Here's how the part is built. I have some questions about the finished solid (model axes, mm). A direction names the side the tool comes from. Give positions to 0.01 mm unless a question says otherwise; leave off trailing zeros. Order: outer loops, then holes, each group sorted by start corner. A loop starts at its lowest first (then second) coordinate and runs counter-clockwise, first axis right, second up. Notation, with made-up numbers: M -1.5,32 L 15.5,32 A24 cw 15.5,55 Z; hole C 40.5,66 d9. An arc over 180 degrees is marked long. Use CSV: the item, a comma, the result in double quotes. Start each with the question number.
```python
from build123d import *

# Parameters (mm, degrees)
PAD028_DEPTH            = 9
SKETCH075_R             = 11.25
POCKET028_DEPTH         = 7
SKETCH076_R             = 8
POCKET029_DEPTH         = 5
SKETCH077_W             = 16
SKETCH077_H             = 37
PAD029_DEPTH            = 9
SKETCH078_W             = 14
SKETCH078_H             = 35
POCKET030_DEPTH         = 1
SKETCH079_W             = 12
SKETCH079_H             = 33
POCKET031_DEPTH         = 5
SKETCH080_W             = 10
SKETCH080_H             = 4
POCKET032_DEPTH         = 5
HOLE007_D               = 4.5
HOLE007_DEPTH           = 25
HOLE007_CBORE_D         = 7.5
HOLE007_CBORE_DEPTH     = 4
FILLET006_R             = 2
BODY010_ROLL_ANGLE      = 180
BODY010_PLACEMENT_ANGLE = -90


with BuildPart() as part:
    # Sketch074 → Pad028 (new body)
    with BuildSketch(Plane.XY):
        with BuildLine():
            ThreePointArc((12.269609, 5), (-13.250782, 0), (12.269609, -5))
            Line((12.269609, -5), (47.729609, -5))
            ThreePointArc((47.729609, -5), (73.25, 0), (47.729609, 5))
            Line((12.269609, 5), (47.729609, 5))
        make_face()
    extrude(amount=PAD028_DEPTH)

    # Sketch075 (on Face6 of Pad028) → Pocket028 (cut)
    with BuildSketch(Plane.XY.offset(9)):
        Circle(SKETCH075_R)
        with Locations((60, 0)):
            Circle(SKETCH075_R)
    extrude(amount=-POCKET028_DEPTH, mode=Mode.SUBTRACT)

    # Sketch076 (on Face4 of Pocket028) → Pocket029 (cut)
    with BuildSketch(Plane(origin=(0, 0, 0), x_dir=(1, 0, 0), z_dir=(0, 0, -1))):
        Circle(SKETCH076_R)
        with Locations((60, 0)):
            Circle(SKETCH076_R)
    extrude(amount=-POCKET029_DEPTH, mode=Mode.SUBTRACT)

    # Sketch077 (on Face4 of Pocket029) → Pad029 (join)
    with BuildSketch(Plane(origin=(0, 0, 0), x_dir=(1, 0, 0), z_dir=(0, 0, -1))):
        with Locations((30, -4.5)):
            Rectangle(SKETCH077_W, SKETCH077_H)
    extrude(amount=-PAD029_DEPTH)

    # Sketch078 (on Face13 of Pad029) → Pocket030 (cut)
    with BuildSketch(Plane.XY.offset(9)):
        with Locations((30, 4.5)):
            Rectangle(SKETCH078_W, SKETCH078_H)
    extrude(amount=-POCKET030_DEPTH, mode=Mode.SUBTRACT)

    # Sketch079 (on Face22 of Pocket030) → Pocket031 (cut)
    with BuildSketch(Plane.XY.offset(9)):
        with Locations((30, 4.5)):
            Rectangle(SKETCH079_W, SKETCH079_H)
    extrude(amount=-POCKET031_DEPTH, mode=Mode.SUBTRACT)

    # Sketch080 (on Face14 of Pocket031) → Pocket032 (cut)
    with BuildSketch(Plane(origin=(0, 23, 0), x_dir=(-1, 0, 0), z_dir=(0, 1, 0))):
        with Locations((-30, 5)):
            Rectangle(SKETCH080_W, SKETCH080_H)
    extrude(amount=-POCKET032_DEPTH, mode=Mode.SUBTRACT)

    # Hole007
    with Locations(Plane(origin=(0, 0, 0), x_dir=(1, 0, 0), z_dir=(0, 0, -1))):
        with Locations((17, 0), (43, 0)):
            CounterBoreHole(HOLE007_D / 2, HOLE007_CBORE_D / 2, HOLE007_CBORE_DEPTH, depth=HOLE007_DEPTH)

    # Fillet006
    fillet006_edges = [part.edges().sort_by_distance(p)[0] for p in [
        (38, 23, 4.5),
        (22, 23, 4.5),
        (22, -14, 4.5),
        (38, -14, 4.5),
    ]]
    fillet(fillet006_edges, radius=FILLET006_R)


with BuildPart() as part_1:
    # Body010 roll: moved
    add(part.part.rotate(Axis((0, 0, 0), (1, 0, 0)), BODY010_ROLL_ANGLE))


with BuildPart() as part_2:
    # Body010 placement: moved
    add(part_1.part.moved(Location((0, 120, 46))).rotate(Axis((0, 120, 46), (0, 0, 1)), BODY010_PLACEMENT_ANGLE))


solid = part_2.part
```
Q1. We'd pull the mould along X, two halves only. Please class faces 6 (the face through (-2, 75, 42)), 7 (the face through (-22, 90, 39)), 8 (the face through (-4, 84, 40)), 9 (the face through (-23, 90, 44)): pulls with the +X half, pulls with the -X half, needs draft (parallel to the pull), parting line crosses it, or undercut.
Q2. I need wall thicknesses on line 1 (Y direction, x = -20, z = 42.25); line 2 (Y direction, x = -0.5, z = 40); line 3 (Y direction, x = -15, z = 38.5). Which ranges of each line are inside material? Lowest first, please. Write a range as [from, to].
Q3. Imagine slicing it at D-D, the plane y = 103. Please give me the cut outline in (x, z).
Q4. For P1, Ø7, axis at x = 0, y = 91.5, coming from the -Z side; P2, Ø1.2, axis at x = -7.5, z = 40, coming from the +Y side; P3, Ø4.5, axis at y = 75.5, z = 41, coming from the -X side, each with a flat end and sliding along its axis, tell me the tip position at first contact or that it passes through.
Q5. Imagine slicing it at B-B, the plane z = 45. Please give me the cut outline in (x, y).
Q6. Imagine slicing it at A-A, the plane y = 60. Please give me the cut outline in (x, z), then the cut area to 3 significant figures.
Q7. Imagine slicing it at C-C, the plane x = -16. Please give me the cut outline in (y, z).
Q8. For faces 1 (the face through (-13, 98, 42)), 2 (the face through (13.4, 97.43, 41.44)), 3 (the face through (-2, 101, 42)), 4 (the face through (-4, 96, 40)), 5 (the face through (-22.43, 82.6, 41.44)), which set-ups out of +Z, -Z, +X, -X, +Y, -Y let a thin tool reach every point of the face, with its end or its side?
Reply:
1,face 6,"undercut"
1,face 7,"needs draft"
1,face 8,"undercut"
1,face 9,"pulls with the -X half"
2,line 1,"y = [82, 85], [95, 98]"
2,line 2,"y = [46.76, 48.76], [71.24, 74.81], [79.19, 84], [96, 100.81], [105.19, 108.76], [131.24, 133.24]"
2,line 3,"y = [82, 84], [96, 98]"
3,outline,"M -5,37 L -2.25,37 L -2.25,42 L -3.75,42 L -3.75,46 L -5,46 Z; M 2.25,37 L 5,37 L 5,46 L 3.75,46 L 3.75,42 L 2.25,42 Z"
4,P1,"stops at z = 42"
4,P2,"stops at y = 131.31"
4,P3,"stops at x = -5"
5,outline,"M -23,84 A2 ccw -21,82 L -5,82 L -5,72.27 A13.25 ccw long 5,72.27 L 5,82 L 12,82 A2 ccw 14,84 L 14,96 A2 ccw 12,98 L 5,98 L 5,107.73 A13.25 ccw long -5,107.73 L -5,98 L -21,98 A2 ccw -23,96 Z; hole C 0,60 d16; hole C 0,120 d16; hole C 0,77 d7.5; hole C 0,103 d7.5"
6,outline,"M -13.25,37 L -11.25,37 L -11.25,44 L -8,44 L -8,46 L -13.25,46 Z; M 8,44 L 11.25,44 L 11.25,37 L 13.25,37 L 13.25,46 L 8,46 Z"
6,area,"49.0 mm^2"
7,outline,"M 82,37 L 83,37 L 83,38 L 84,38 L 84,42 L 96,42 L 96,38 L 97,38 L 97,37 L 98,37 L 98,46 L 82,46 Z"
8,face 1,"+Z, -Z, -X"
8,face 2,"+Z, -Z, +X"
8,face 3,"+Z"
8,face 4,"-Z"
8,face 5,"+Z, -Z, -X, -Y"
